from build123d import *

# Parameters (mm, degrees)
SKETCH1_W           = 7.62
SKETCH1_H           = 4.8768
BOSS_EXTRUDE1_DEPTH = 17.78
BOSS_EXTRUDE2_DEPTH = 32.385
CUT_EXTRUDE1_DEPTH  = 8.62
SKETCH5_R           = 2.54
BOSS_EXTRUDE3_DEPTH = 3.048
SKETCH7_R           = 2.286
BOSS_EXTRUDE4_DEPTH = 2.54


with BuildPart() as part:
    # Sketch1 → Boss-Extrude1 (new body, symmetric)
    with BuildSketch(Plane(origin=(0, 0, 0), x_dir=(0, 0, -1), z_dir=(1, 0, 0))):
        Rectangle(SKETCH1_W, SKETCH1_H)
    extrude(amount=BOSS_EXTRUDE1_DEPTH, both=True)

    # Sketch2 → Boss-Extrude2 (add)
    with BuildSketch(Plane(origin=(17.78, 0, 0), x_dir=(0, 0, -1), z_dir=(1, 0, 0))):
        Polygon((-3.4925, 3.9116), (3.4925, 3.9116), (2.3495, 2.4384), (-2.3495, 2.4384), align=None)
    extrude(amount=-BOSS_EXTRUDE2_DEPTH)

    # Sketch3 → Cut-Extrude1 (cut, through all)
    with BuildSketch(Plane.XY.offset(3.81)):
        Polygon((17.78, -2.4384), (15.494, 3.9116), (17.78, 3.9116), align=None)
    extrude(amount=-CUT_EXTRUDE1_DEPTH, mode=Mode.SUBTRACT)

    # Sketch5 → Boss-Extrude3 (add)
    with BuildSketch(Plane.XY.offset(3.81)):
        with Locations((-13.0175, 0.7366)):
            Circle(SKETCH5_R)
    boss_extrude3 = extrude(amount=BOSS_EXTRUDE3_DEPTH)

    # Sketch7 → Boss-Extrude4 (add)
    with BuildSketch(Plane.XY.offset(6.858)):
        with Locations((-13.0175, 0.7366)):
            Circle(SKETCH7_R)
    boss_extrude4 = extrude(amount=BOSS_EXTRUDE4_DEPTH)

    # Mirror1: Boss-Extrude3, Boss-Extrude4 across plane
    add(boss_extrude3.mirror(Plane.XY))
    add(boss_extrude4.mirror(Plane.XY))


solid = part.part
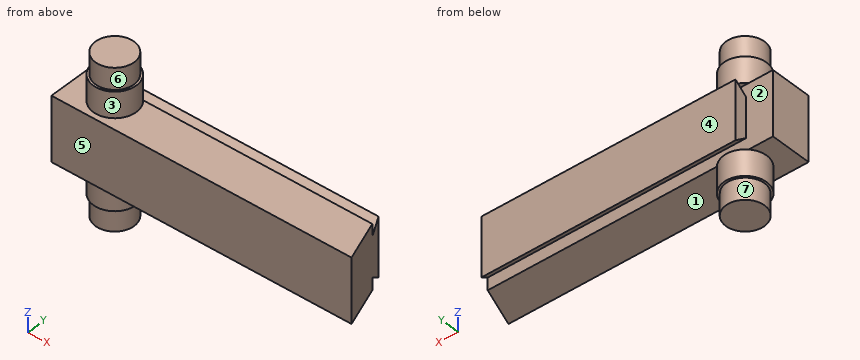
For this review, take the finished solid that the model builds, in its own axes (mm). Face numbers are marked on the shaded views. A direction names the side the tool comes from. Give positions to 0.01 mm unless a question says otherwise; leave off trailing zeros. Loops run counter-clockwise (first coordinate to the right, second up) from the corner with the lowest first, then second, coordinate; pieces in that order, holes last. Notation, with made-up numbers: M 56,53.25 L 72,53.25 A11 ccw 72,69.25 Z; hole C 58.25,49 d2. An arc over 180 degrees is marked long. Put each result on its own line as item: value. Start each with the question number.
(1) Add section C-C, the plane z = -2. Write out the cut boundary in (x, y) (3 decimals), then the cut area to 3 significant figures.
(2) Add section A-A, the plane x = 14.5. Write out the cut boundary in (y, z), then the cut area to 3 significant figures.
(3) For pin 1 (1.2 mm diameter, centred on y = 3.5, z = 0.5, fed in from -X) (3 decimals); pin 2 (1 mm diameter, centred on x = -0.5, y = -1.5, fed in from +Z); pin 3 (1 mm diameter, centred on x = 14, y = 1.5, fed in from -Z), all flat-tipped, find the tip position at first contact; note any pin that passes through.
(4) Add section B-B, the plane y = 2. Write out the cut boundary in (x, z), then the cut area to 3 significant figures.
(5) The part is to be moulded in two halves that separate along Y. For the marked faces 1, 2, 3 and 4, say which applies: +Y half, -Y half, draft (parallel to the pull), parting line (faces both ways), or undercut.
(6) Machinability: for the marked faces 5, 6 and 7, which of the approach directions +Z, -Z, +X, -X, +Y, -Y give a long, thin tool a straight path to every point of the face, cutting with its end or side? Answer none if there is none.
(7) Add section D-D, the plane x = -14. Write out the cut boundary in (y, z).
(8) Wall thickness on L1, parallel to Z at x = 6, y = 0.75; L2, parallel to Y at x = -2, z = 3.75; L3, parallel to Y at x = 15, z = 2.5: over which ranges is each line inside the solid? List them lowest first.
Result:
1. outline: M -17.78,-2.438 L 17.78,-2.438 L 15.494,3.912 L -14.605,3.912 L -14.605,2.438 L -17.78,2.438 Z
1. area: 214 mm^2
2. outline: M -2.44,-3.81 L 2.44,-3.81 L 2.44,-2.35 L 3.91,-3.49 L 3.91,3.49 L 2.44,2.35 L 2.44,3.81 L -2.44,3.81 Z
2. area: 45.8 mm^2
3. pin 1: stops at x = -14.605
3. pin 2: stops at z = 3.81
3. pin 3: stops at z = -3.81
4. outline: M -17.78,-3.81 L -15.22,-3.81 L -15.22,-6.86 L -14.92,-6.86 L -14.92,-9.4 L -11.11,-9.4 L -11.11,-6.86 L -10.81,-6.86 L -10.81,-3.81 L 16.18,-3.81 L 16.18,3.81 L -10.81,3.81 L -10.81,6.86 L -11.11,6.86 L -11.11,9.4 L -14.92,9.4 L -14.92,6.86 L -15.22,6.86 L -15.22,3.81 L -17.78,3.81 Z
4. area: 305 mm^2
5. face 1: draft
5. face 2: undercut
5. face 3: parting line
5. face 4: +Y half
6. face 5: +Z, -Z, +X, -X, -Y
6. face 6: +Z
6. face 7: -Z
7. outline: M -2.44,-3.81 L -1.61,-3.81 L -1.61,-6.86 L -1.33,-6.86 L -1.33,-9.4 L 2.8,-9.4 L 2.8,-6.86 L 3.08,-6.86 L 3.08,-3.81 L 2.44,-3.81 L 2.44,-2.35 L 3.91,-3.49 L 3.91,3.49 L 2.44,2.35 L 2.44,3.81 L 3.08,3.81 L 3.08,6.86 L 2.8,6.86 L 2.8,9.4 L -1.33,9.4 L -1.33,6.86 L -1.61,6.86 L -1.61,3.81 L -2.44,3.81 Z
8. L1: z = -3.81 to 3.81
8. L2: y = -2.44 to 2.44
8. L3: y = -2.44 to 2.44, 2.63 to 3.91
